Design review of the part built by this model. Coordinates are the model's own, in mm. Coordinates: 2 decimals unless noted, no trailing zeros. Write each loop counter-clockwise with the first axis right and the second up, starting at its lowest first coordinate (ties: lowest second). Pieces come first, ordered by that corner, then holes.
Q1. Clearance check with flat-ended pins moving along their axes: pin 1 Ø1.4 at (x, y) = (6, 4) entering from -Z; pin 2 Ø0.6 at (x, z) = (5, 12.5) entering from -Y; pin 3 Ø5 at (x, z) = (5.5, 21) entering from -Y; pin 4 Ø1.7 at (y, z) = (2, 18.5) entering from -X. State where each tip first meets the part, or that it passes through.
Q2. Add section C-C, the plane y = 1.75. Give the boundary of the cut face in (x, z), plus the area to 3 significant figures.
Q3. Add section B-B, the plane y = 4. Give the number of separate pieces and of enclosed holes in the cut face, plus the area to 3 significant figures.
Q4. To check wall thickness, follow probe 1 along Y at (x, z) = (-2, 24.75); probe 2 along Y at (x, z) = (2.5, 19); probe 3 along Y at (x, z) = (-1.5, 21.5). State the ranges of each line that lie inside material, in increasing order.
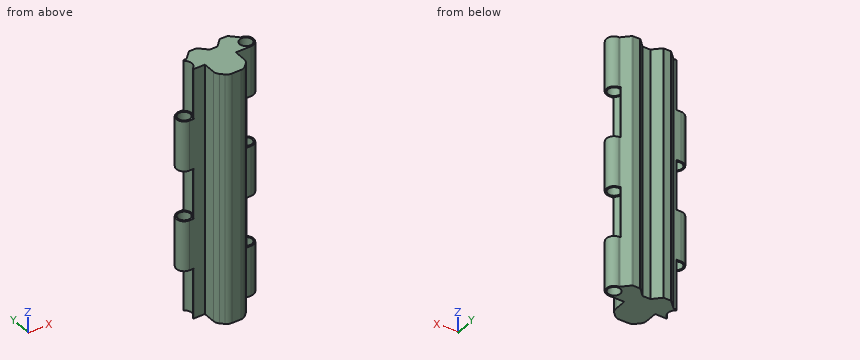
from build123d import *

# Parameters (mm, degrees)
BOSS_EXTRUDE1_DEPTH  = 32.5
CHAMFER1_SIZE        = 1
FILLET1_R            = 1
BOSS_EXTRUDE7_DEPTH  = 32.5
SKETCH3_R            = 0.9999999999999979
BOSS_EXTRUDE9_DEPTH  = 6.5
LPATTERN2_COUNT      = 3
LPATTERN2_PITCH      = 13
SKETCH5_R            = 1.0000000000000002
BOSS_EXTRUDE10_DEPTH = 6.5
LPATTERN3_COUNT      = 2
LPATTERN3_PITCH      = 13
FILLET2_R            = 0.1
M2_TAPPED_HOLE1_D    = 1.6
FILLET3_R            = 0.1


with BuildPart() as part:
    # Sketch1 → Boss-Extrude1 (new body)
    with BuildSketch(Plane.XY):
        Polygon((0, 0), (4, 0), (3.9999999999999982, 4), (-1.73e-15, 4), align=None)
    extrude(amount=BOSS_EXTRUDE1_DEPTH)

    # Chamfer1
    chamfer1_edges = [part.edges().sort_by_distance(p)[0] for p in [
        (4, 0, 16.25),
        (0, 0, 16.25),
    ]]
    chamfer(chamfer1_edges, length=CHAMFER1_SIZE)

    # Fillet1
    fillet1_edges = [part.edges().sort_by_distance(p)[0] for p in [
        (3, 0, 16.25),
        (1, 0, 16.25),
        (-4.3e-16, 1, 16.25),
        (3.9999999999999996, 1, 16.25),
    ]]
    fillet(fillet1_edges, radius=FILLET1_R)

    # Sketch2 → Boss-Extrude7 (add)
    with BuildSketch(Plane.XY.offset(32.5)):
        with BuildLine():
            Line((-1.73e-15, 3), (-2, 2.9999999999999996))
            ThreePointArc((-2, 2.9999999999999996), (-1.0000000000000009, 4), (-2, 4.999999999999999))
            Line((-2, 4.999999999999999), (-1.0000000000000009, 4.999999999999999))
            Line((-1.0000000000000009, 4.999999999999999), (-1.74e-15, 6.000000000000002))
            Line((-1.74e-15, 6.000000000000002), (1, 6))
            Line((1, 6), (2.000000000000004, 4.999999999999999))
            Line((2.000000000000004, 4.999999999999999), (3.000000000000002, 4.999999999999997))
            Line((3.000000000000002, 4.999999999999997), (4.000000000000002, 6))
            Line((4.000000000000002, 6), (5.0000000000000036, 5.999999999999998))
            Line((5.0000000000000036, 5.999999999999998), (6.000000000000008, 4.999999999999997))
            ThreePointArc((6.000000000000008, 4.999999999999997), (5.000000000000009, 3.9999999999999982), (6.000000000000008, 3))
            Line((6.000000000000008, 3), (-1.73e-15, 3))
        make_face()
    extrude(amount=-BOSS_EXTRUDE7_DEPTH)

    # Sketch3 → Boss-Extrude9 (add)
    with BuildSketch(Plane.XY.offset(32.5)):
        with Locations((6.000000000000008, 3.9999999999999982)):
            Circle(SKETCH3_R)
    boss_extrude9 = extrude(amount=-BOSS_EXTRUDE9_DEPTH)

    # LPattern2: Boss-Extrude9 ×3
    with Locations(*[(0, 0, -i * LPATTERN2_PITCH) for i in range(1, LPATTERN2_COUNT)]):
        add(boss_extrude9)

    # Sketch5 → Boss-Extrude10 (add)
    with BuildSketch(Plane.XY.offset(26.000000000000004)):
        with Locations((-2, 4)):
            Circle(SKETCH5_R)
    boss_extrude10 = extrude(amount=-BOSS_EXTRUDE10_DEPTH)

    # LPattern3: Boss-Extrude10 ×2
    with Locations(*[(0, 0, -i * LPATTERN3_PITCH) for i in range(1, LPATTERN3_COUNT)]):
        add(boss_extrude10)

    # Fillet2
    fillet2_edges = [part.edges().sort_by_distance(p)[0] for p in [
        (6.000000000000008, 4.999999999999998, 9.75),
        (6.000000000000008, 3, 9.75),
        (-2, 4.999999999999999, 29.25),
        (-2, 2.9999999999999996, 29.25),
        (-2, 4.999999999999999, 16.250000000000004),
        (-2, 2.9999999999999996, 16.250000000000004),
        (-2, 2.9999999999999996, 3.25),
        (-2, 4.999999999999999, 3.25),
        (6.000000000000008, 4.999999999999998, 22.75),
        (6.000000000000008, 3, 22.75),
    ]]
    fillet(fillet2_edges, radius=FILLET2_R)

    # M2 Tapped Hole1 (through all)
    with Locations(Plane(origin=(0, 0, 0), x_dir=(-1, 0, 0), z_dir=(0, 0, -1))):
        with Locations((-6, 4), (2, 4)):
            Hole(M2_TAPPED_HOLE1_D / 2)

    # Fillet3
    fillet3_edges = [part.edges().sort_by_distance(p)[0] for p in [
        (6.000000000000008, 4.999999999999998, 3.25),
        (-1.0000000000000009, 4.999999999999999, 16.25),
        (-1.74e-15, 6.000000000000002, 16.25),
        (1, 6, 16.25),
        (2.000000000000004, 4.999999999999999, 16.25),
        (3.000000000000002, 4.999999999999997, 16.25),
        (4.000000000000002, 6, 16.25),
        (5.0000000000000036, 5.999999999999998, 16.25),
        (6.000000000000008, 4.999999999999998, 29.25),
        (6.000000000000008, 4.999999999999998, 16.25),
    ]]
    fillet(fillet3_edges, radius=FILLET3_R)


solid = part.part
Here are the results:
1. pin 1: passes through
1. pin 2: stops at y = 3
1. pin 3: stops at y = 0.09
1. pin 4: stops at x = 0
2. outline: (0, 0) - (4, 0) - (4, 32.5) - (0, 32.5) - close
2. area: 130 mm2
3. separate pieces: 6
3. enclosed holes: 0
3. area: 208 mm2
4. probe 1: y = 3 to 3.2, 4.8 to 5
4. probe 2: y = 0 to 5
4. probe 3: y = 3 to 3.38, 4.62 to 5
